from build123d import *
from build123d.topology import SkipClean

# Parameters (mm, degrees)
BOSS_EXTRUDE1_DEPTH = 2.5
BOSS_EXTRUDE2_DEPTH = 22
BOSS_EXTRUDE3_DEPTH = 3
CUT_EXTRUDE1_DEPTH  = 24.5
BOSS_EXTRUDE4_START = 32.5
BOSS_EXTRUDE4_DEPTH = 32.5
FILLET1_R           = 1.3


with BuildPart() as part:
    # Sketch1 → Boss-Extrude1 (new body)
    with BuildSketch(Plane.XY.offset(27.5)):
        with BuildLine():
            Line((-1.7, 0), (-1.7, -2.01))
            ThreePointArc((-1.7, -2.01), (-0.728058535, -3.546206617), (1.076389141, -3.325821575))
            Line((1.076389141, -3.325821575), (2.613987517, -2.068011074))
            Line((2.613987517, -2.068011074), (2.613987517, 0.214645493))
            Line((2.613987517, 0.214645493), (0.99224156, 1.380382804))
            ThreePointArc((0.99224156, 1.380382804), (-0.775625344, 1.512747608), (-1.7, 0))
        make_face()
        with BuildLine():
            Line((0.679355547, -0.590318593), (0.679355547, -1.419681407))
            ThreePointArc((0.679355547, -1.419681407), (-0.315103164, -1.166963823), (-0.9, -2.01))
            Line((-0.9, -2.01), (-0.9, 0))
            ThreePointArc((-0.9, 0), (-0.315103164, -0.843036177), (0.679355547, -0.590318593))
        make_face(mode=Mode.SUBTRACT)
        with BuildLine():
            Line((1.630572559, -1.838904922), (0.569853074, -2.706611422))
            ThreePointArc((0.569853074, -2.706611422), (0.854555431, -2.292373892), (0.872712282, -1.79006075))
            Line((0.872712282, -1.79006075), (0.923994115, -1.764796557))
            ThreePointArc((0.923994115, -1.764796557), (1.261831892, -1.949170927), (1.630572559, -1.838904922))
        make_face(mode=Mode.SUBTRACT)
        with BuildLine():
            Line((0.525304355, 0.730790896), (1.60582327, -0.045903634))
            ThreePointArc((1.60582327, -0.045903634), (1.206195872, 0.036344151), (0.878343375, -0.206512796))
            Line((0.878343375, -0.206512796), (0.876200076, -0.205605026))
            ThreePointArc((0.876200076, -0.205605026), (0.842771024, 0.315811655), (0.525304355, 0.730790896))
        make_face(mode=Mode.SUBTRACT)
        with BuildLine():
            Line((1.813987517, -0.451898576), (1.813987517, -1.451898576))
            ThreePointArc((1.813987517, -1.451898576), (1.699848532, -1.133918581), (1.409542408, -0.961114242))
            Line((1.409542408, -0.961114242), (1.412543995, -0.942088969))
            ThreePointArc((1.412543995, -0.942088969), (1.700819677, -0.768696431), (1.813987517, -0.451898576))
        make_face(mode=Mode.SUBTRACT)
    extrude(amount=-BOSS_EXTRUDE1_DEPTH)

    # Sketch2 → Boss-Extrude2 (add)
    with BuildSketch(Plane(origin=(0, 0, 25), x_dir=(-1, 0, 0), z_dir=(0, 0, -1))):
        with BuildLine():
            Line((-0.872712282, -1.79006075), (-0.923994115, -1.764796557))
            ThreePointArc((-0.923994115, -1.764796557), (-1.741947592, -1.710452584), (-1.409542408, -0.961114242))
            Line((-1.409542408, -0.961114242), (-1.412543995, -0.942088968))
            ThreePointArc((-1.412543995, -0.942088968), (-1.718555312, -0.158087582), (-0.878343375, -0.206512796))
            Line((-0.878343375, -0.206512796), (-0.876200076, -0.205605026))
            ThreePointArc((-0.876200076, -0.205605026), (0.801211243, 0.40995188), (-0.679355547, -0.590318593))
            Line((-0.679355547, -0.590318593), (-0.679355547, -1.419681407))
            ThreePointArc((-0.679355547, -1.419681407), (0.797824448, -2.426504681), (-0.872712282, -1.79006075))
        make_face()
    extrude(amount=BOSS_EXTRUDE2_DEPTH)

    # Sketch3 → Boss-Extrude3 (add)
    with BuildSketch(Plane(origin=(0, 0, 3), x_dir=(-1, 0, 0), z_dir=(0, 0, -1))):
        with BuildLine():
            Line((-0.679355547, -0.590318593), (-0.679355547, -1.419681407))
            ThreePointArc((-0.679355547, -1.419681407), (0.828144816, -2.362386385), (-0.896420024, -1.929805603))
            ThreePointArc((-0.896420024, -1.929805603), (-1.576433756, -2.029721828), (-1.948619488, -1.451898576))
            Line((-1.948619488, -1.451898576), (-1.948619488, -0.451898576))
            ThreePointArc((-1.948619488, -0.451898576), (-1.578314183, 0.125066892), (-0.8995417, 0.028718114))
            ThreePointArc((-0.8995417, 0.028718114), (0.847956803, 0.301611107), (-0.679355547, -0.590318593))
        make_face()
    extrude(amount=BOSS_EXTRUDE3_DEPTH)

    # Sketch4 → Cut-Extrude1 (cut)
    with BuildSketch(Plane.XY.offset(27.5)):
        with BuildLine():
            Line((0.679355547, -0.590318593), (0.679355547, -1.419681407))
            ThreePointArc((0.679355547, -1.419681407), (0.747780209, -1.50917592), (0.804488538, -1.60651742))
            Line((0.804488538, -1.60651742), (0.833948407, -1.591764415))
            ThreePointArc((0.833948407, -1.591764415), (0.881698314, -1.200649606), (1.197901281, -0.965561259))
            Line((1.197901281, -0.965561259), (1.197901281, -0.938235893))
            ThreePointArc((1.197901281, -0.938235893), (0.900174078, -0.732537913), (0.819207563, -0.379837516))
            Line((0.819207563, -0.379837516), (0.816593613, -0.378384554))
            ThreePointArc((0.816593613, -0.378384554), (0.755443566, -0.489188122), (0.679355547, -0.590318593))
        make_face()
    extrude(amount=-CUT_EXTRUDE1_DEPTH, mode=Mode.SUBTRACT)

    # Sketch5 → Boss-Extrude4 (add)
    with SkipClean():  # the faces are left unmerged after this step: merging them gives an invalid solid
        with BuildSketch(Plane.XY.offset(27.5).offset(BOSS_EXTRUDE4_START)):
            with BuildLine():
                Line((0.923994116, -1.764796557), (0.872712282, -1.79006075))
                ThreePointArc((0.872712282, -1.79006075), (-0.84360695, -2.323571865), (0.804488538, -1.60651742))
                Line((0.804488538, -1.60651742), (0.833948407, -1.591764415))
                ThreePointArc((0.833948407, -1.591764415), (0.881698314, -1.200649606), (1.197901281, -0.965561259))
                Line((1.197901281, -0.965561259), (1.197901281, -0.938235893))
                ThreePointArc((1.197901281, -0.938235893), (0.900174078, -0.732537913), (0.819207563, -0.379837516))
                Line((0.819207563, -0.379837516), (0.816593613, -0.378384554))
                ThreePointArc((0.816593613, -0.378384554), (-0.850794223, 0.293511823), (0.876200076, -0.205605026))
                Line((0.876200076, -0.205605026), (0.878343375, -0.206512796))
                ThreePointArc((0.878343375, -0.206512796), (1.718555312, -0.158087582), (1.412543995, -0.942088968))
                Line((1.412543995, -0.942088968), (1.409542408, -0.961114242))
                ThreePointArc((1.409542408, -0.961114242), (1.741947592, -1.710452584), (0.923994116, -1.764796557))
            make_face()
        extrude(amount=-BOSS_EXTRUDE4_DEPTH)

    # Fillet1
    fillet1_edges = [part.edges().sort_by_distance(p)[0] for p in [
        (2.613987517, 0.214645493, 26.25),
        (2.613987517, -2.068011074, 26.25),
    ]]
    fillet(fillet1_edges, radius=FILLET1_R)


solid = part.part
Design review of the part built by this model. Coordinates are the model's own, in mm. A direction names the side the tool comes from. Coordinates: 2 decimals unless noted, no trailing zeros. Loops run counter-clockwise (first coordinate to the right, second up) from the corner with the lowest first, then second, coordinate; pieces in that order, holes last.
Item 1: For faces 5 (the flat face through (1.814, -1, 26)), 6 (the flat face through (1.949, -1, 2)), 7 (the flat face through (2, -1, 27.5)), list the 3-axis set-ups (+Z, -Z, +X, -X, +Y, -Y) from which the entire face can be reached by the end or side of a thin tool; tool diameter is ignored.
Completed:
face 5: none
face 6: -Z, +X, +Y, -Y
face 7: +Z
Item 2: Add section A-A (x = 0). Write out the cut boundary in (y, z), and give its area (3 significant figures).
Completed:
outline: (-3.71, 25) - (-2.91, 25) - (-2.91, 0) - (-1.11, 0) - (-1.11, 60) - (-2.91, 60) - (-2.91, 27.5) - (-3.71, 27.5) - close; (-0.9, 0) - (0.9, 0) - (0.9, 25) - (1.7, 25) - (1.7, 27.5) - (0.9, 27.5) - (0.9, 60) - (-0.9, 60) - close
area: 220 mm2
Item 3: Draft analysis for pull direction X (two halves, no side actions). For faces 1 (the flat face through (-1.7, -1, 26)), 2 (the flat face through (0.48, -0.55, 60)), 3 (the flat face through (1.6, -2.9, 26.3)), 4 (the flat face through (1.058, 0.348, 26.268)), state which applies: pulls with the +X half, pulls with the -X half, needs draft (parallel to the pull), parting line crosses it, or undercut.
Completed:
face 1: pulls with the -X half
face 2: needs draft
face 3: pulls with the +X half
face 4: undercut
Item 4: Wall thickness on L1, parallel to Y at x = -0.1, z = 16; L2, parallel to Z at x = 2.15, y = -0.05; L3, parallel to Y at x = -0.3, z = 11: over which ranges is each line inside the solid? List them lowest first.
Completed:
L1: y = -2.9 to -1.12, -0.89 to 0.89
L2: z = 25 to 27.5
L3: y = -2.86 to -1.16, -0.85 to 0.85
Item 5: Clearance check with flat-ended pins moving along their axes: pin 1 (2 mm diameter, centred on y = -3, z = 15.5, fed in from -X); pin 2 (0.8 mm diameter, centred on y = -1, z = 2, fed in from +X); pin 3 (1.5 mm diameter, centred on y = -2.5, z = 33.5, fed in from +X). State where each tip first meets the part, or that it passes through.
Completed:
pin 1: stops at x = -0.9
pin 2: stops at x = 1.95
pin 3: stops at x = 1.72
